from build123d import *

# Parameters (mm, degrees)
SKETCH1_W            = 240
SKETCH1_H            = 240
BOSS_EXTRUDE1_DEPTH  = 4
M5_CLEARANCE_HOLE1_D = 5.5
M3_CLEARANCE_HOLE1_D = 3.4


with BuildPart() as part:
    # Sketch1 → Boss-Extrude1 (new body)
    with BuildSketch(Plane(origin=(0, 0, 0), x_dir=(1, 0, 0), z_dir=(0, 1, 0))):
        with Locations((100, 100)):
            Rectangle(SKETCH1_W, SKETCH1_H)
    extrude(amount=BOSS_EXTRUDE1_DEPTH)

    # M5 Clearance Hole1 (through all)
    with Locations(Plane(origin=(0, 4, 0), x_dir=(1, 0, 0), z_dir=(0, 1, 0))):
        with Locations((18.682720164, 181.317279836), (181.436841233, 181.317279836), (181.436841233, 18.3), (18.682720164, 18.3), (40, 210), (100, 210), (160, 210), (210, 160), (210, 100), (210, 40), (160, -10), (100, -10), (40, -10), (-10, 40), (-10, 100), (-10, 157.735112715), (94.988544792, 157.28119514), (47.887302245, 124.30055005), (105.011455208, 42.71880486), (147.101242547, 132.98064509), (152.112697755, 75.69944995), (52.898757453, 67.01935491), (77.5, 100), (122.5, 100)):
            Hole(M5_CLEARANCE_HOLE1_D / 2)

    # M3 Clearance Hole1 (through all)
    with Locations(Plane(origin=(0, 4, 0), x_dir=(1, 0, 0), z_dir=(0, 1, 0))):
        with Locations((37.378342924, 144.00490984), (76.440621755, 163.90813502), (66.861094929, 134.425383015)):
            Hole(M3_CLEARANCE_HOLE1_D / 2)


solid = part.part
Build history of the part. All positions in model axes, mm. Round coordinates to 2 decimals unless told otherwise and drop trailing zeros. Write each loop counter-clockwise with the first axis right and the second up, starting at its lowest first coordinate (ties: lowest second). Pieces come first, ordered by that corner, then holes. Notation, with made-up numbers: M -33.5,71.5 L -4.5,71.5 A9 ccw -4.5,82.5 Z; hole C 78,64.5 d4. An arc over 180 degrees is marked long. Answer as a JSON object with one key per item and string values. Group by question number.
(1) Flat gauge pin, fed straight in: pin 1 (5 mm diameter, centred on x = 181.44, z = -18.3, fed in from +Y). Where does the tip first touch, or does it go through?
(2) Mould opens along X. For faces 1 (the flat face through (98, 0, -102)), 2 (the cylindrical face through (147.5, 2, -135.7)) say: pulls with the +X half, pulls with the -X half, needs draft (parallel to the pull), parting line crosses it, or undercut.
(3) Cut at B-B (x = 122.5). Give the cut face in (y, z).
(4) Drill centre lines: L1, parallel to X at y = 1.35, z = -18.3; L2, parallel to Z at x = 40, y = 1.3; L3, parallel to X at y = 0.9, z = -39.5. Where is each one in solid material? Low to high.
(5) Cut at A-A (z = -210). Give the cut face in (x, y).
Responses:
{
 "1": {"pin 1": "passes through"},
 "2": {"face 1": "needs draft", "face 2": "undercut"},
 "3": {"outline": "M 0,-220 L 4,-220 L 4,-102.75 L 0,-102.75 Z; M 0,-97.25 L 4,-97.25 L 4,20 L 0,20 Z"},
 "4": {"L1": "x = -20 to 15.93, 21.43 to 178.69, 184.19 to 220", "L2": "z = -220 to -212.75, -207.25 to 7.25, 12.75 to 20", "L3": "x = -20 to -12.7, -7.3 to 207.3, 212.7 to 220"},
 "5": {"outline": "M -20,0 L 37.25,0 L 37.25,4 L -20,4 Z; M 42.75,0 L 97.25,0 L 97.25,4 L 42.75,4 Z; M 102.75,0 L 157.25,0 L 157.25,4 L 102.75,4 Z; M 162.75,0 L 220,0 L 220,4 L 162.75,4 Z"}
}
